```python
from build123d import *

# Parameters (mm, degrees)
SKETCH2_R                    = 150
SKETCH2_R_2                  = 65
BOSS_EXTRUDE1_DEPTH          = 15
TAP_DRILL_FOR_M14X2_0_TAP1_D = 20
CIRPATTERN1_COUNT            = 6
TAP_DRILL_FOR_M14X2_0_TAP2_D = 18
CIRPATTERN2_COUNT            = 2


with BuildPart() as part:
    # Sketch2 → Boss-Extrude1 (new body)
    with BuildSketch(Plane(origin=(0, 0, 0), x_dir=(1, 0, 0), z_dir=(0, 1, 0))):
        Circle(SKETCH2_R)
        Circle(SKETCH2_R_2, mode=Mode.SUBTRACT)
    extrude(amount=BOSS_EXTRUDE1_DEPTH)

    # Tap Drill for M14x2.0 Tap1 (through all)
    with Locations(Plane(origin=(0, 15, 0), x_dir=(1, 0, 0), z_dir=(0, 1, 0))):
        with Locations((0, 120)):
            tap_drill_for_m14x2_0_tap1 = Hole(TAP_DRILL_FOR_M14X2_0_TAP1_D / 2)

    # CirPattern1: Tap Drill for M14x2.0 Tap1 ×6 about axis
    cirpattern1_axis = Axis((0, 0, 0), (0, 1, 0))
    for i in range(1, CIRPATTERN1_COUNT):
        add(tap_drill_for_m14x2_0_tap1.rotate(cirpattern1_axis, i * 360 / CIRPATTERN1_COUNT), mode=Mode.SUBTRACT)

    # Tap Drill for M14x2.0 Tap2 (through all)
    with Locations(Plane(origin=(0, 15, 0), x_dir=(1, 0, 0), z_dir=(0, 1, 0))):
        with Locations((0, 80)):
            tap_drill_for_m14x2_0_tap2 = Hole(TAP_DRILL_FOR_M14X2_0_TAP2_D / 2)

    # CirPattern2: Tap Drill for M14x2.0 Tap2 ×2 about axis
    cirpattern2_axis = Axis((0, 0, 0), (0, 1, 0))
    for i in range(1, CIRPATTERN2_COUNT):
        add(tap_drill_for_m14x2_0_tap2.rotate(cirpattern2_axis, i * 360 / CIRPATTERN2_COUNT), mode=Mode.SUBTRACT)


solid = part.part
```
Model file for the job. Use its own axes, mm. Coordinates: 2 decimals unless noted, no trailing zeros. Loops run counter-clockwise (first coordinate to the right, second up) from the corner with the lowest first, then second, coordinate; pieces in that order, holes last. Notation, with made-up numbers: (84.25, 2) - (104.25, 2) arc R6 cw to (104.25, 13) - close; hole circle Ø10 at (-21.75, 83.25). An arc over 180 degrees is marked (long way). Answer as a JSON object with one key per item and string values. Group by question number.
(1) Flat gauge pins, fed straight in: pin 1 (5 mm diameter, centred on y = 13.5, z = -94, fed in from -X); pin 2 (6 mm diameter, centred on x = -91.5, y = 1.5, fed in from +Z); pin 3 (3 mm diameter, centred on y = 9, z = -105, fed in from -X). Where does each tip first touch, or does it go through?
(2) Cut at C-C (y = 10.5). State how many separate pieces and enclosed holes the cut face has, then the cut area to 3 significant figures.
(3) Probe line 1 along Z through (x, y) = (0, 7.5); line 2 along Z through (x, y) = (-96, 11.5); line 3 along X through (y, z) = (8.25, -60). List the from-to ranges inside material, lowest first.
(4) Cut at B-B (x = -54). Give the cut face in (y, z), then the cut area to 3 significant figures.
(5) Cut at A-A (z = 120). Give the cut face in (x, y).
(6) Two-plate mould, pull along X, no slides. Class faces 1 (the face through (65, 15, 31)), 2 (the face through (-113.461, 7.395, 56.996)), 3 (the face through (-19.527, 7.395, -148.724)): released by +X, released by -X, zero draft, split by the parting line, or undercut.
(7) Cut at D-D (z = -60). Give the cut face in (x, y).
Geometry says:
{
 "1": {"pin 1": "stops at x = -118.86", "pin 2": "stops at z = 121.11", "pin 3": "stops at x = -108.57"},
 "2": {"separate pieces": "1", "enclosed holes": "9", "area": "55,000 mm^2"},
 "3": {"line 1": "z = -150 to -130, -110 to -89, -71 to -65, 65 to 71, 89 to 110, 130 to 150", "line 2": "z = -115.26 to -66.1, -53.9 to 53.9, 66.1 to 115.26", "line 3": "x = -137.48 to -113.92, -93.92 to -25, 25 to 93.92, 113.92 to 137.48"},
 "4": {"outline": "(0, -139.94) - (15, -139.94) - (15, -36.18) - (0, -36.18) - close; (0, 36.18) - (15, 36.18) - (15, 139.94) - (0, 139.94) - close", "area": "3,110 mm^2"},
 "5": {"outline": "(-90, 0) - (-10, 0) - (-10, 15) - (-90, 15) - close; (10, 0) - (90, 0) - (90, 15) - (10, 15) - close"},
 "6": {"face 1": "zero draft", "face 2": "undercut", "face 3": "split by the parting line"},
 "7": {"outline": "(-137.48, 0) - (-113.92, 0) - (-113.92, 15) - (-137.48, 15) - close; (-93.92, 0) - (-25, 0) - (-25, 15) - (-93.92, 15) - close; (25, 0) - (93.92, 0) - (93.92, 15) - (25, 15) - close; (113.92, 0) - (137.48, 0) - (137.48, 15) - (113.92, 15) - close"}
}
